from build123d import *

# Parameters (mm, degrees)
SKETCH_1_W          = 17.893001423
SKETCH_1_H          = 11.620982588
SKETCH_1_H_2        = 11.620982589
EXTRUDE_1_DEPTH     = 1
SKETCH_2_R          = 1.5
CUT_EXTRUDE_1_DEPTH = 10
SKETCH_3_R          = 1.5
CUT_EXTRUDE_2_DEPTH = 10
SKETCH_4_W          = 33.892879225
SKETCH_4_H          = 96
CUT_EXTRUDE_3_DEPTH = 10


with BuildPart() as part:
    # Эскиз1 → Бобышка-Вытянуть1 (new body)
    with BuildSketch(Plane(origin=(0, 0, 0), x_dir=(1, 0, 0), z_dir=(0, 1, 0))):
        Polygon((49.933797981, 26), (18.809932441, 26), (18.809932441, 48), (15, 48), (-48.959081244, 48), (-48.959081244, -48), (15, -48), (18.809932441, -48), (18.809932441, -26), (49.933797981, -26), align=None)
        with Locations((-36.319088007, -31.12001489)):
            Rectangle(SKETCH_1_W, SKETCH_1_H, mode=Mode.SUBTRACT)
        with Locations((-36.319088007, 31.12001489)):
            Rectangle(SKETCH_1_W, SKETCH_1_H_2, mode=Mode.SUBTRACT)
    extrude(amount=EXTRUDE_1_DEPTH)

    # Эскиз2 → Вырез-Вытянуть1 (cut)
    with BuildSketch(Plane(origin=(0, 1, 0), x_dir=(1, 0, 0), z_dir=(0, 1, 0))):
        with Locations(Location((46.183797981, -14.4, 0), (0, 0, 270))):
            Circle(SKETCH_2_R)
        with Locations(Location((18.683797981, -14.4, 0), (0, 0, 270))):
            Circle(SKETCH_2_R)
        with Locations(Location((18.683797981, -4.4, 0), (0, 0, 270))):
            Circle(SKETCH_2_R)
        with Locations(Location((46.183797981, -4.4, 0), (0, 0, 270))):
            Circle(SKETCH_2_R)
        with Locations(Location((18.683797981, 5.6, 0), (0, 0, 270))):
            Circle(SKETCH_2_R)
        with Locations(Location((46.183797981, 5.6, 0), (0, 0, 270))):
            Circle(SKETCH_2_R)
        with Locations(Location((18.683797981, 15.6, 0), (0, 0, 270))):
            Circle(SKETCH_2_R)
        with Locations(Location((46.183797981, 15.6, 0), (0, 0, 270))):
            Circle(SKETCH_2_R)
    extrude(amount=-CUT_EXTRUDE_1_DEPTH, mode=Mode.SUBTRACT)

    # Эскиз3 → Вырез-Вытянуть2 (cut)
    with BuildSketch(Plane(origin=(0, 1, 0), x_dir=(1, 0, 0), z_dir=(0, 1, 0))):
        with Locations(Location((5.923569009, 32.746976788, 0), (0, 0, 270))):
            Circle(SKETCH_3_R)
        with Locations(Location((-2.726430991, 32.746976788, 0), (0, 0, 270))):
            Circle(SKETCH_3_R)
        with Locations(Location((-2.726430991, -35.660220789, 0), (0, 0, 270))):
            Circle(SKETCH_3_R)
        with Locations(Location((5.923569009, -35.660220789, 0), (0, 0, 270))):
            Circle(SKETCH_3_R)
    extrude(amount=-CUT_EXTRUDE_2_DEPTH, mode=Mode.SUBTRACT)

    # Эскиз4 → Вырез-Вытянуть3 (cut)
    with BuildSketch(Plane.XZ):
        with Locations((-32.012641632, 0)):
            Rectangle(SKETCH_4_W, SKETCH_4_H)
    extrude(amount=-CUT_EXTRUDE_3_DEPTH, mode=Mode.SUBTRACT)


solid = part.part
Design review of the part built by this model. Coordinates are the model's own, in mm. Coordinates: 2 decimals unless noted, no trailing zeros. Loops run counter-clockwise (first coordinate to the right, second up) from the corner with the lowest first, then second, coordinate; pieces in that order, holes last. Notation, with made-up numbers: M 86.25,-29 L 110.25,-29 A5 ccw 110.25,-20 Z; hole C 66,74.5 d2. An arc over 180 degrees is marked long. Use one line per item in the form item = value.
(1) Consider section C-C (x = 42.5). Write out the cut boundary in (y, z), and give its area (3 significant figures).
Return value:
outline = M 0,-26 L 1,-26 L 1,26 L 0,26 Z
area = 52.0 mm2
(2) Consider section B-B (y = 0.4). Give the number of separate pieces and of enclosed holes in the cut face, and give its area (3 significant figures).
Return value:
separate_pieces = 1
enclosed_holes = 12
area = 4,790 mm2
(3) Clearance check with flat-ended pins moving along their axes: P1, Ø8, axis at x = 16, z = -15.5, coming from the -Y side; P2, Ø0.5, axis at y = 0.5, z = -34, coming from the +X side. State where each tip first meets the part, or that it passes through.
Return value:
P1 = 0
P2 = 18.81
(4) Consider section A-A (z = 4.4). Write out the cut boundary in (x, y), and give its area (3 significant figures).
Return value:
outline = M -15.07,0 L 17.18,0 L 17.18,1 L -15.07,1 Z; M 20.18,0 L 44.68,0 L 44.68,1 L 20.18,1 Z; M 47.68,0 L 49.93,0 L 49.93,1 L 47.68,1 Z
area = 59.0 mm2
(5) Consider section D-D (z = 32.5). Write out the cut boundary in (x, y), and give its area (3 significant figures).
Return value:
outline = M -15.07,0 L 18.81,0 L 18.81,1 L -15.07,1 Z
area = 33.9 mm2
(6) Draft analysis for pull direction Y (two halves, no side actions). For faces 1 (the face through (10, 1, -1)), 2 (the face through (10, 0, -1)), 3 (the face through (47.67, 0.51, -5.8)), state which applies: pulls with the +Y half, pulls with the -Y half, needs draft (parallel to the pull), parting line crosses it, or undercut.
Return value:
face_1 = pulls with the +Y half
face_2 = pulls with the -Y half
face_3 = needs draft
(7) For line 1 along X through (y, z) = (0.5, 4.4); line 2 along Z through (x, y) = (-4, 0.3); line 3 along Z through (x, y) = (47.5, 0.65), list the stretches that pass through material, from the lowest coordinate up. Write a range as from..to.
Return value:
line_1 = -15.07..17.18, 20.18..44.68, 47.68..49.93
line_2 = -48..-33.54, -31.95..34.87, 36.45..48
line_3 = -26..-16.32, -14.88..-6.32, -4.88..3.68, 5.12..13.68, 15.12..26
